Check sheet for the modelled part. Datum: model origin and axes. Units: mm. Coordinates: 2 decimals unless noted, no trailing zeros. Order: outer loops, then holes, each group sorted by start corner. A loop starts at its lowest first (then second) coordinate and runs counter-clockwise, first axis right, second up.
from build123d import *

# Parameters (mm, degrees)
SKETCH1_W                 = 120
SKETCH1_H                 = 100
BOSS_EXTRUDE1_DEPTH       = 2.9718
SKETCH2_W                 = 70
SKETCH2_H                 = 20
CUT_EXTRUDE1_DEPTH        = 3.9718
SKETCH3_W                 = 29.908
SKETCH3_H                 = 3.048
CUT_EXTRUDE2_DEPTH        = 3.9718
SKETCH4_W                 = 10
SKETCH4_H                 = 20
SKETCH4_W_2               = 2.54
SKETCH4_H_2               = 6.604
CUT_EXTRUDE3_DEPTH        = 2.9718
MIRROR2_COPY_1_SKETCH_W   = 29.908
MIRROR2_COPY_1_SKETCH_H   = 3.048
MIRROR2_COPY_1_DEPTH      = 3.9718
MIRROR2_COPY_2_SKETCH_W   = 10
MIRROR2_COPY_2_SKETCH_H   = 20
MIRROR2_COPY_2_SKETCH_W_2 = 2.54
MIRROR2_COPY_2_SKETCH_H_2 = 6.604
MIRROR2_COPY_2_DEPTH      = 2.9718
SKETCH6_W                 = 50
SKETCH6_H                 = 11.0236
CUT_EXTRUDE4_DEPTH        = 3.9718
SKETCH7_W                 = 30
SKETCH7_H                 = 11.0236
CUT_EXTRUDE6_DEPTH        = 3.9718
SKETCH8_R                 = 1.524
CUT_EXTRUDE7_DEPTH        = 3.9718
SKETCH11_R                = 1.524
CUT_EXTRUDE8_DEPTH        = 3.9718


with BuildPart() as part:
    # Sketch1 → Boss-Extrude1 (new body)
    with BuildSketch(Plane(origin=(0, 0, 0), x_dir=(1, 0, 0), z_dir=(0, 1, 0))):
        Rectangle(SKETCH1_W, SKETCH1_H)
    extrude(amount=BOSS_EXTRUDE1_DEPTH)

    # Sketch2 → Cut-Extrude1 (cut, through all)
    with BuildSketch(Plane(origin=(0, 2.9718, 0), x_dir=(1, 0, 0), z_dir=(0, 1, 0))):
        with Locations((0, 50)):
            Rectangle(SKETCH2_W, SKETCH2_H)
    extrude(amount=-CUT_EXTRUDE1_DEPTH, mode=Mode.SUBTRACT)

    # Sketch3 → Cut-Extrude2 (cut, through all)
    with BuildSketch(Plane(origin=(0, 2.9718, 0), x_dir=(1, 0, 0), z_dir=(0, 1, 0))):
        with Locations((-60, 20)):
            Rectangle(SKETCH3_W, SKETCH3_H)
    cut_extrude2 = extrude(amount=-CUT_EXTRUDE2_DEPTH, mode=Mode.SUBTRACT)

    # Sketch4 → Cut-Extrude3 (cut)
    with BuildSketch(Plane(origin=(0, 2.9718, 0), x_dir=(1, 0, 0), z_dir=(0, 1, 0))):
        with Locations((-60, 20)):
            Rectangle(SKETCH4_W, SKETCH4_H)
        with Locations((-50.046, 20)):
            Rectangle(SKETCH4_W_2, SKETCH4_H_2)
    cut_extrude3 = extrude(amount=-CUT_EXTRUDE3_DEPTH, mode=Mode.SUBTRACT)

    # Mirror1: Cut-Extrude2, Cut-Extrude3 across plane
    add(cut_extrude2.mirror(Plane.XY), mode=Mode.SUBTRACT)
    add(cut_extrude3.mirror(Plane.XY), mode=Mode.SUBTRACT)

    # Mirror2: Cut-Extrude3, Cut-Extrude2 across plane
    add(cut_extrude3.mirror(Plane(origin=(0, 0, 0), x_dir=(0, 0, 1), z_dir=(1, 0, 0))), mode=Mode.SUBTRACT)
    add(cut_extrude2.mirror(Plane(origin=(0, 0, 0), x_dir=(0, 0, 1), z_dir=(1, 0, 0))), mode=Mode.SUBTRACT)

    # Mirror2 copy 1 sketch → Mirror2 copy 1 (cut, through all)
    with BuildSketch(Plane(origin=(0, 2.9718, 0), x_dir=(-1, 0, 0), z_dir=(0, 1, 0))):
        with Locations((-60, 20)):
            Rectangle(MIRROR2_COPY_1_SKETCH_W, MIRROR2_COPY_1_SKETCH_H)
    extrude(amount=-MIRROR2_COPY_1_DEPTH, mode=Mode.SUBTRACT)

    # Mirror2 copy 2 sketch → Mirror2 copy 2 (cut)
    with BuildSketch(Plane(origin=(0, 2.9718, 0), x_dir=(-1, 0, 0), z_dir=(0, 1, 0))):
        with Locations((-60, 20)):
            Rectangle(MIRROR2_COPY_2_SKETCH_W, MIRROR2_COPY_2_SKETCH_H)
        with Locations((-50.046, 20)):
            Rectangle(MIRROR2_COPY_2_SKETCH_W_2, MIRROR2_COPY_2_SKETCH_H_2)
    extrude(amount=-MIRROR2_COPY_2_DEPTH, mode=Mode.SUBTRACT)

    # Sketch6 → Cut-Extrude4 (cut, through all)
    with BuildSketch(Plane(origin=(0, 2.9718, 0), x_dir=(1, 0, 0), z_dir=(0, 1, 0))):
        with Locations((-60, -50)):
            Rectangle(SKETCH6_W, SKETCH6_H)
        with Locations((60, -50)):
            Rectangle(SKETCH6_W, SKETCH6_H)
    extrude(amount=-CUT_EXTRUDE4_DEPTH, mode=Mode.SUBTRACT)

    # Sketch7 → Cut-Extrude6 (cut, through all)
    with BuildSketch(Plane(origin=(0, 2.9718, 0), x_dir=(1, 0, 0), z_dir=(0, 1, 0))):
        with Locations((0, -50)):
            Rectangle(SKETCH7_W, SKETCH7_H)
    extrude(amount=-CUT_EXTRUDE6_DEPTH, mode=Mode.SUBTRACT)

    # Sketch8 → Cut-Extrude7 (cut, through all)
    with BuildSketch(Plane(origin=(0, 2.9718, 0), x_dir=(1, 0, 0), z_dir=(0, 1, 0))):
        with Locations((-25, -46.0122)):
            Circle(SKETCH8_R)
        with Locations((25, -46.0122)):
            Circle(SKETCH8_R)
    extrude(amount=-CUT_EXTRUDE7_DEPTH, mode=Mode.SUBTRACT)

    # Sketch11 → Cut-Extrude8 (cut, through all)
    with BuildSketch(Plane(origin=(0, 2.9718, 0), x_dir=(1, 0, 0), z_dir=(0, 1, 0))):
        with Locations((-56.2474, 0)):
            Circle(SKETCH11_R)
        with Locations((56.2474, 0)):
            Circle(SKETCH11_R)
    extrude(amount=-CUT_EXTRUDE8_DEPTH, mode=Mode.SUBTRACT)


solid = part.part
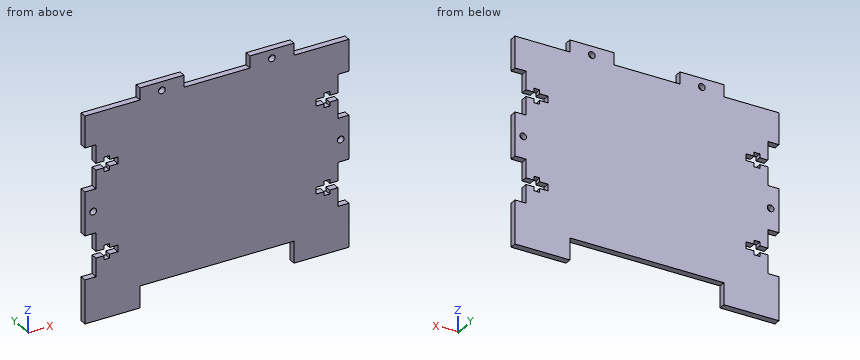
(1) Cross-section at C-C (x = 9.5). Enter the section's corners in (y, z).
Filled in:
outline: (0, -40) - (2.97, -40) - (2.97, 44.49) - (0, 44.49) - close
(2) Thickness scan on probe 1 along X at (y, z) = (2.05, 0); probe 2 along Z at (x, y) = (53.5, 2.85); probe 3 along Z at (x, y) = (25, 0.7). Record the ranges inside material, lowest first.
Filled in:
probe 1: x = -60 to -57.77, -54.72 to 54.72, 57.77 to 60
probe 2: z = -50 to -21.52, -18.48 to 18.48, 21.52 to 44.49
probe 3: z = -40 to 44.49, 47.54 to 50
(3) Go/stop test with flat-tipped pins: P1, Ø0.9, axis at y = 1.5, z = 26, coming from the -X side; P2, Ø1.3, axis at x = 49.5, y = 1.5, coming from the +Z side; P3, Ø1, axis at x = 32, y = 1, coming from the -Z side. Record where each tip stops, or that it passes through.
Filled in:
P1: stops at x = -55
P2: stops at z = 44.49
P3: stops at z = -40
(4) Cross-section at A-A (z = 0). Enter the section's corners in (x, y).
Filled in:
outline: (-60, 0) - (-57.77, 0) - (-57.77, 2.97) - (-60, 2.97) - close; (-54.72, 0) - (54.72, 0) - (54.72, 2.97) - (-54.72, 2.97) - close; (57.77, 0) - (60, 0) - (60, 2.97) - (57.77, 2.97) - close
(5) Cross-section at B-B (x = -25). Enter the section's corners in (y, z).
Filled in:
outline: (0, -40) - (2.97, -40) - (2.97, 44.49) - (0, 44.49) - close; (0, 47.54) - (2.97, 47.54) - (2.97, 50) - (0, 50) - close
(6) Cross-section at D-D (y = 0.6). Count the separate pieces of the cut face and the enclosed holes in it, and give its area (3 significant figures).
Filled in:
separate pieces: 1
enclosed holes: 4
area: 10,300 mm2
